from build123d import *

# Parameters (mm, degrees)
SKETCH_1_R          = 38
SKETCH_1_R_2        = 30
EXTRUDE_1_DEPTH     = 8
SKETCH_2_R          = 35.25
SKETCH_2_R_2        = 31.75
CUT_EXTRUDE_1_DEPTH = 1
SKETCH_3_R          = 35.25
SKETCH_3_R_2        = 31.75
CUT_EXTRUDE_2_DEPTH = 1


with BuildPart() as part:
    # 草图1 → 凸台-拉伸1 (new body)
    with BuildSketch(Plane(origin=(0, 0, 0), x_dir=(1, 0, 0), z_dir=(0, 1, 0))):
        Circle(SKETCH_1_R)
        Circle(SKETCH_1_R_2, mode=Mode.SUBTRACT)
    extrude(amount=EXTRUDE_1_DEPTH)

    # 草图2 → 切除-拉伸1 (cut)
    with BuildSketch(Plane(origin=(0, 8, 0), x_dir=(1, 0, 0), z_dir=(0, 1, 0))):
        Circle(SKETCH_2_R)
        Circle(SKETCH_2_R_2, mode=Mode.SUBTRACT)
    extrude(amount=-CUT_EXTRUDE_1_DEPTH, mode=Mode.SUBTRACT)

    # 草图3 → 切除-拉伸2 (cut)
    with BuildSketch(Plane.XZ):
        Circle(SKETCH_3_R)
        Circle(SKETCH_3_R_2, mode=Mode.SUBTRACT)
    extrude(amount=-CUT_EXTRUDE_2_DEPTH, mode=Mode.SUBTRACT)


solid = part.part
Read the model definition and answer for the solid it produces. Units are mm, in the model's axes. A direction names the side the tool comes from. Round coordinates to 2 decimals unless told otherwise and drop trailing zeros. Loops run counter-clockwise (first coordinate to the right, second up) from the corner with the lowest first, then second, coordinate; pieces in that order, holes last.
Q1. Each of these flat-tipped pins is pushed along its axis until it touches: pin 1 (5 mm diameter, centred on x = 24, z = -21, fed in from +Y); pin 2 (2 mm diameter, centred on x = 10, y = 7, fed in from +Z); pin 3 (6 mm diameter, centred on x = -0.5, z = -24, fed in from +Y); pin 4 (1 mm diameter, centred on y = 4, z = -25.5, fed in from +X). Where does it stop, or does it pass through?
Q2. Which of the six approach directions +Z, -Z, +X, -X, +Y, -Y give full straight-line access (tool end or side, diameter ignored) to faces 5 (the face through (28, 0, 12)), 6 (the face through (-27.97, 0.49, -21.45)), 7 (the face through (-31.5, 7, -5.4))?
Q3. Section B-B on x = 0 is taken. Write down the section's boundary in (y, z).
Q4. Section A-A on z = 0 is taken. Write down the section's boundary in (x, y).
Q5. Section C-C on y = 3 is taken. Write down the section's boundary in (x, z), and give its area (3 significant figures).
Q6. Consider probe 1 along X at (y, z) = (7.75, 0); probe 2 along X at (y, z) = (7.25, -25). Determine where each line is inside the solid, lowest interval first.
Q7. Determine the mould class of faces 1 (the face through (-31.5, 1, 5.4)), 2 (the face through (-6.883, 7.507, 30.995)), 3 (the face through (17.535, 3.944, 33.713)), 4 (the face through (11, 0, 34)) for opening direction X: released by +X, released by -X, zero draft, split by the parting line, or undercut.
Output:
1. pin 1: stops at y = 8
1. pin 2: stops at z = 36.92
1. pin 3: passes through
1. pin 4: stops at x = 28.62
2. face 5: +Z, -Z, +X, -X, -Y
2. face 6: -Y
2. face 7: +Y
3. outline: (0, -38) - (8, -38) - (8, -35.25) - (7, -35.25) - (7, -31.75) - (8, -31.75) - (8, -30) - (0, -30) - (0, -31.75) - (1, -31.75) - (1, -35.25) - (0, -35.25) - close; (0, 30) - (8, 30) - (8, 31.75) - (7, 31.75) - (7, 35.25) - (8, 35.25) - (8, 38) - (0, 38) - (0, 35.25) - (1, 35.25) - (1, 31.75) - (0, 31.75) - close
4. outline: (-38, 0) - (-35.25, 0) - (-35.25, 1) - (-31.75, 1) - (-31.75, 0) - (-30, 0) - (-30, 8) - (-31.75, 8) - (-31.75, 7) - (-35.25, 7) - (-35.25, 8) - (-38, 8) - close; (30, 0) - (31.75, 0) - (31.75, 1) - (35.25, 1) - (35.25, 0) - (38, 0) - (38, 8) - (35.25, 8) - (35.25, 7) - (31.75, 7) - (31.75, 8) - (30, 8) - close
5. outline: circle Ø76 at (0, 0); hole circle Ø60 at (0, 0)
5. area: 1,710 mm2
6. probe 1: x = -38 to -35.25, -31.75 to -30, 30 to 31.75, 35.25 to 38
6. probe 2: x = -28.62 to -24.85, -19.57 to -16.58, 16.58 to 19.57, 24.85 to 28.62
7. face 1: undercut
7. face 2: undercut
7. face 3: split by the parting line
7. face 4: zero draft
